Here's how the part is built. I have some questions about the finished solid (model axes, mm). Face numbers are marked on the shaded views. A direction names the side the tool comes from. Coordinates: 2 decimals unless noted, no trailing zeros. Order: outer loops, then holes, each group sorted by start corner. A loop starts at its lowest first (then second) coordinate and runs counter-clockwise, first axis right, second up. Notation, with made-up numbers: M 83.5,-20.75 L 142.5,-20.75 A23 cw 142.5,-8.75 Z; hole C 47,42.5 d5. An arc over 180 degrees is marked long. One line per question, with ' | ' between items. Start each with the question number.
```python
from build123d import *

# Parameters (mm, degrees)
SKETCH1_R           = 65
BOSS_EXTRUDE1_DEPTH = 3
SKETCH2_R           = 3
CUT_EXTRUDE1_DEPTH  = 4
CIRPATTERN1_COUNT   = 4
SKETCH3_R           = 65
SKETCH3_R_2         = 60
BOSS_EXTRUDE2_DEPTH = 40
SKETCH4_R           = 20
BOSS_EXTRUDE3_DEPTH = 40
SKETCH5_R           = 10
CUT_EXTRUDE2_DEPTH  = 30
SKETCH6_R           = 1
CUT_EXTRUDE3_DEPTH  = 44


with BuildPart() as part:
    # Sketch1 → Boss-Extrude1 (new body)
    with BuildSketch(Plane(origin=(0, 0, 0), x_dir=(1, 0, 0), z_dir=(0, 1, 0))):
        Circle(SKETCH1_R)
    extrude(amount=BOSS_EXTRUDE1_DEPTH)

    # Sketch2 → Cut-Extrude1 (cut, through all)
    with BuildSketch(Plane(origin=(0, 3, 0), x_dir=(1, 0, 0), z_dir=(0, 1, 0))):
        with Locations((0, 55)):
            Circle(SKETCH2_R)
    cut_extrude1 = extrude(amount=-CUT_EXTRUDE1_DEPTH, mode=Mode.SUBTRACT)

    # CirPattern1: Cut-Extrude1 ×4 about axis
    cirpattern1_axis = Axis((0, 0, 0), (0, 1, 0))
    for i in range(1, CIRPATTERN1_COUNT):
        add(cut_extrude1.rotate(cirpattern1_axis, i * 360 / CIRPATTERN1_COUNT), mode=Mode.SUBTRACT)

    # Sketch3 → Boss-Extrude2 (add)
    with BuildSketch(Plane(origin=(0, 3, 0), x_dir=(1, 0, 0), z_dir=(0, 1, 0))):
        Circle(SKETCH3_R)
        Circle(SKETCH3_R_2, mode=Mode.SUBTRACT)
    extrude(amount=BOSS_EXTRUDE2_DEPTH)

    # Sketch4 → Boss-Extrude3 (add)
    with BuildSketch(Plane(origin=(0, 3, 0), x_dir=(1, 0, 0), z_dir=(0, 1, 0))):
        Circle(SKETCH4_R)
    extrude(amount=BOSS_EXTRUDE3_DEPTH)

    # Sketch5 → Cut-Extrude2 (cut)
    with BuildSketch(Plane.XZ):
        Circle(SKETCH5_R)
    extrude(amount=-CUT_EXTRUDE2_DEPTH, mode=Mode.SUBTRACT)

    # Sketch6 → Cut-Extrude3 (cut, through all)
    with BuildSketch(Plane(origin=(0, 43, 0), x_dir=(1, 0, 0), z_dir=(0, 1, 0))):
        Circle(SKETCH6_R)
    extrude(amount=-CUT_EXTRUDE3_DEPTH, mode=Mode.SUBTRACT)


solid = part.part
```
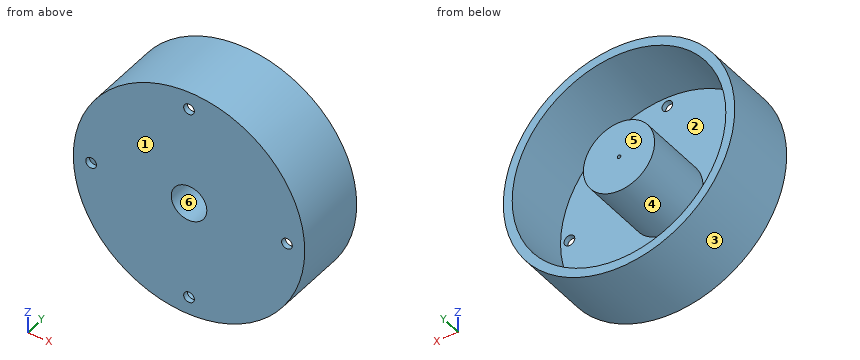
1. Will these pins go through, and if not, where does the flat tip stop? pin 1 (8 mm diameter, centred on x = 0, z = -55, fed in from +Y); pin 2 (6 mm diameter, centred on x = -4, z = 1.5, fed in from -Y); pin 3 (1 mm diameter, centred on y = 28, z = 21.5, fed in from -X); pin 4 (2.5 mm diameter, centred on x = 0, z = 0, fed in from +Y).
2. Imagine slicing it at B-B (x = -45.5). List the corners of the cut face in (y, z) for me, then the cut area to 3 significant figures.
3. I need wall thicknesses on line 1 (Z direction, x = 0, y = 0.7); line 2 (X direction, y = 39, z = 0); line 3 (Z direction, x = 0, y = 6.25). Which ranges of each line are inside material? Lowest first, please.
4. Imagine slicing it at D-D (x = 39). List the corners of the cut face in (y, z) for me, then the cut area to 3 significant figures.
5. Imagine slicing it at A-A (y = 26). List the corners of the cut face in (x, z) for me, then the cut area to 3 significant figures.
6. Which directions (+Z, -Z, +X, -X, +Y, -Y) give clear straight access to the entire face, cutting with the end or side of a thin tool? Please do the marked faces 4, 5 and 6.
7. Imagine slicing it at C-C (z = 55). List the corners of the cut face in (x, y) for me.
8. We'd pull the mould along X, two halves only. Please class the marked faces 1, 2 and 3: released by +X, released by -X, zero draft, split by the parting line, or undercut.
Entries:
1) pin 1: y = 3 | pin 2: y = 30 | pin 3: x = -61.51 | pin 4: y = 43
2) outline: M 0,-46.42 L 43,-46.42 L 43,-39.11 L 3,-39.11 L 3,39.11 L 43,39.11 L 43,46.42 L 0,46.42 Z | area: 863 mm²
3) line 1: -65 to -58, -52 to -10, 10 to 52, 58 to 65 | line 2: -65 to -60, -20 to -1, 1 to 20, 60 to 65 | line 3: -65 to -60, -20 to -10, 10 to 20, 60 to 65
4) outline: M 0,-52 L 43,-52 L 43,-45.6 L 3,-45.6 L 3,45.6 L 43,45.6 L 43,52 L 0,52 Z | area: 824 mm²
5) outline: C 0,0 d130; C 0,0 d40; hole C 0,0 d120; hole C 0,0 d20 | area: 2,910 mm²
6) face 4: +Y | face 5: +Z, -Z, +X, -X, +Y | face 6: -Y
7) outline: M -34.64,0 L -3,0 L -3,3 L -23.98,3 L -23.98,43 L -34.64,43 Z; M 3,0 L 34.64,0 L 34.64,43 L 23.98,43 L 23.98,3 L 3,3 Z
8) face 1: zero draft | face 2: undercut | face 3: split by the parting line
